Source: CAD feature listing. Evaluate the final solid. Frame: model axes, mm. Face numbers are marked on the shaded views. Give positions to 0.01 mm unless a question says otherwise; leave off trailing zeros. Loops run counter-clockwise (first coordinate to the right, second up) from the corner with the lowest first, then second, coordinate; pieces in that order, holes last.
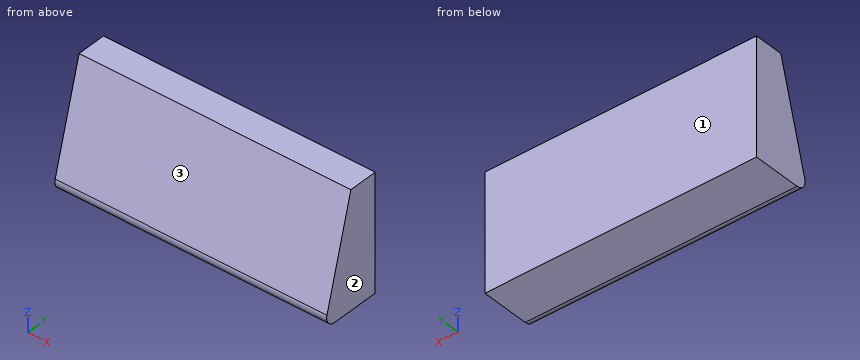
```python
from build123d import *

# Parameters (mm, degrees)
PAD_DEPTH = 14


with BuildPart() as part:
    # Sketch → Pad (new body, symmetric)
    with BuildSketch(Plane.YZ):
        with BuildLine():
            Line((0, 0), (0, 12))
            Line((0, 12), (-3, 12))
            Line((-3, 12), (-5.963927, 1.266168))
            ThreePointArc((-5.963927, 1.266168), (-5.795666, 0.394264), (-5, 0))
            Line((-5, 0), (0, 0))
        make_face()
    extrude(amount=PAD_DEPTH, both=True)


solid = part.part
```
(1) First-contact query: pin 1 (2 mm diameter, centred on x = 4, z = 2.5, fed in from -Y). Flat tip, straight axial feed; report the tip coordinate or a pass-through.
A:
pin 1: stops at y = -5.9
(2) Section B-B, the plane z = 3. Return the cut outline in (x, y), then the cut area to 3 significant figures.
A:
outline: (-14, -5.49) - (14, -5.49) - (14, 0) - (-14, 0) - close
area: 154 mm2
(3) Ray query, line 1 along Y through (x, z) = (3.5, 1.25); line 2 along Y through (x, z) = (8.5, 6). Return the intervals inside material, ascending.
A:
line 1: y = -5.97 to 0
line 2: y = -4.66 to 0
(4) Section C-C, the plane y = -5.5. Return the cut outline in (x, z), then the cut area to 3 significant figures.
A:
outline: (-14, 0.13) - (14, 0.13) - (14, 2.95) - (-14, 2.95) - close
area: 78.7 mm2
(5) Mould query, pull axis Y, two halves, no side actions, for the marked faces 1, 2 and 3. Classes: pulls with the +Y half, pulls with the -Y half, needs draft (parallel to the pull), parting line crosses it, or undercut.
A:
face 1: pulls with the +Y half
face 2: needs draft
face 3: pulls with the -Y half
(6) Section A-A, the plane x = -9.5. Return the cut outline in (y, z).
A:
outline: (-5.96, 1.27) arc R1 ccw to (-5, 0) - (0, 0) - (0, 12) - (-3, 12) - close
